from build123d import *

# Parameters (mm, degrees)
BOSS_EXTRUDE1_DEPTH        = 36.33
SKETCH2_R                  = 12.56
SKETCH2_R_2                = 9.25
BOSS_EXTRUDE2_DEPTH        = 20.17
SKETCH3_R                  = 13.815
BOSS_EXTRUDE3_DEPTH        = 20.35
BOSS_EXTRUDE4_DEPTH        = 47.86
CUT_EXTRUDE1_DEPTH         = 8.000000034
SKETCH6_R                  = 6.5
CUT_EXTRUDE2_DEPTH         = 86.564913353
SKETCH7_R                  = 3.8
BOSS_EXTRUDE5_DEPTH        = 17.8
F_10_32_TAPPED_HOLE1_D     = 4.0386
F_10_32_TAPPED_HOLE1_DEPTH = 17.8


with BuildPart() as part:
    # Sketch1 → Boss-Extrude1 (new body)
    with BuildSketch(Plane(origin=(0, 0, 0), x_dir=(1, 0, 0), z_dir=(0, 1, 0))):
        with BuildLine():
            Line((-25, 15), (-25, -15))
            ThreePointArc((-25, -15), (-0.303555948, -21.362892261), (25, -18.18))
            Line((25, -18.18), (25, 18.18))
            ThreePointArc((25, 18.18), (-0.303555948, 21.362892261), (-25, 15))
        make_face()
    extrude(amount=-BOSS_EXTRUDE1_DEPTH)

    # Sketch2 → Boss-Extrude2 (add)
    with BuildSketch(Plane(origin=(25, 0, 0), x_dir=(0, 0, -1), z_dir=(1, 0, 0))):
        with Locations((0, -18.165)):
            Circle(SKETCH2_R)
        with Locations((0, -18.165)):
            Circle(SKETCH2_R_2, mode=Mode.SUBTRACT)
    extrude(amount=BOSS_EXTRUDE2_DEPTH)

    # Sketch3 → Boss-Extrude3 (add)
    with BuildSketch(Plane.XZ.offset(36.33)):
        with Locations(Location((-1.315, 0, 0), (0, 0, 270))):
            Circle(SKETCH3_R)
    extrude(amount=BOSS_EXTRUDE3_DEPTH)

    # Sketch4 → Boss-Extrude4 (add)
    with BuildSketch(Plane(origin=(25, 0, 0), x_dir=(0, 0, -1), z_dir=(1, 0, 0))):
        Polygon((-9.13, -66), (-9.13, -53.08), (9.13, -53.08), (9.13, -66), (4.07, -71.38), (-4.07, -71.38), align=None)
    extrude(amount=-BOSS_EXTRUDE4_DEPTH)

    # Sketch5 → Cut-Extrude1 (cut)
    with BuildSketch(Plane(origin=(25, 0, 0), x_dir=(0, 0, -1), z_dir=(1, 0, 0))):
        Polygon((-9.13, -66), (-4.07, -71.38), (4.07, -71.38), (9.13, -66), (9.13, -53.08), (-9.13, -53.08), align=None)
    extrude(amount=-CUT_EXTRUDE1_DEPTH, mode=Mode.SUBTRACT)

    # Sketch6 → Cut-Extrude2 (cut, through all)
    with BuildSketch(Plane(origin=(16.999999966, 0, 0), x_dir=(0, 0, -1), z_dir=(1, 0, 0))):
        with Locations((0, -61.881671093)):
            Circle(SKETCH6_R)
    extrude(amount=-CUT_EXTRUDE2_DEPTH, mode=Mode.SUBTRACT)

    # Sketch7 → Boss-Extrude5 (add)
    with BuildSketch(Plane.XZ.offset(71.38)):
        with Locations(Location((-13.64, 12.01, 0), (0, 0, 270))):
            Circle(SKETCH7_R)
        with Locations(Location((8.41, -12.01, 0), (0, 0, 270))):
            Circle(SKETCH7_R)
    extrude(amount=-BOSS_EXTRUDE5_DEPTH)

    # #10-32 Tapped Hole1
    with Locations(Plane(origin=(0, -71.38, 0), x_dir=(-1, 0, 0), z_dir=(0, -1, 0))):
        with Locations((13.64, -12.01), (-8.41, 12.01)):
            Hole(F_10_32_TAPPED_HOLE1_D / 2, depth=F_10_32_TAPPED_HOLE1_DEPTH)


solid = part.part
Check sheet for the modelled part. Datum: model origin and axes. Units: mm. A direction names the side the tool comes from. Give positions to 0.01 mm unless a question says otherwise; leave off trailing zeros. Order: outer loops, then holes, each group sorted by start corner. A loop starts at its lowest first (then second) coordinate and runs counter-clockwise, first axis right, second up. Notation, with made-up numbers: (9, 38) - (42, 38) arc R23 cw to (42, 60) - close; hole circle Ø3 at (80.5, 33.25). An arc over 180 degrees is marked (long way). Answer as CSV lines item,"result".
1. Section check C-C (x = -13.64). Record the boundary of the cut face in (y, z).
Result sheet:
outline,"(-71.38, -4.07) - (-66, -9.13) - (-53.08, -9.13) - (-53.08, -6.24) - (-36.33, -6.24) - (-36.33, -19.17) - (0, -19.17) - (0, 19.17) - (-36.33, 19.17) - (-36.33, 6.24) - (-53.08, 6.24) - (-53.08, 9.13) - (-53.58, 9.13) - (-53.58, 9.99) - (-71.38, 9.99) - (-71.38, 8.21) - (-66.98, 8.21) - (-71.38, 4.07) - close; (-71.38, 14.03) - (-53.58, 14.03) - (-53.58, 15.81) - (-71.38, 15.81) - close; hole circle Ø13 at (-61.88, 0)"
2. Mould release check, pull along X, two halves, no side actions. Record for faces 1 (the face through (-11.714, -62.355, 11.403)), 2 (the face through (-25, -18, 0)), 3 (the face through (25, -18, 0)): released by +X, released by -X, zero draft, split by the parting line, or undercut.
Result sheet:
face 1,"undercut"
face 2,"released by -X"
face 3,"released by +X"
3. Section check D-D (z = -5). Record the boundary of the cut face in (x, y).
Result sheet:
outline,"(-25, -36.33) - (-14.19, -36.33) - (-14.19, -53.08) - (-22.86, -53.08) - (-22.86, -57.73) - (17, -57.73) - (17, -53.08) - (11.56, -53.08) - (11.56, -36.33) - (25, -36.33) - (25, -29.69) - (45.17, -29.69) - (45.17, -25.95) - (25, -25.95) - (25, -10.38) - (45.17, -10.38) - (45.17, -6.64) - (25, -6.64) - (25, 0) - (-25, 0) - close; (-22.86, -70.39) - (17, -70.39) - (17, -66.03) - (-22.86, -66.03) - close"
4. Section check B-B (x = 14). Record the boundary of the cut face in (y, z), then the cut area to 3 significant figures.
Result sheet:
outline,"(-71.38, -4.07) - (-66, -9.13) - (-53.08, -9.13) - (-53.08, 9.13) - (-66, 9.13) - (-71.38, 4.07) - close; (-36.33, -20.76) - (0, -20.76) - (0, 20.76) - (-36.33, 20.76) - close; hole circle Ø13 at (-61.88, 0)"
area,"1,680 mm²"
5. Scan lines: probe 1 along Y at (x, z) = (-21.5, 0.5); probe 2 along X at (y, z) = (-64, 12.01); probe 3 along Z at (x, y) = (-13.64, -60.75). Record each from-to range of solid material in increasing order. Write a range as from..to.
Result sheet:
probe 1,"-71.38..-68.36, -55.4..-53.08, -36.33..0"
probe 2,"-17.44..-15.66, -11.62..-9.84"
probe 3,"-9.13..-6.4, 6.4..9.99, 14.03..15.81"
6. Section check A-A (z = 0). Record the boundary of the cut face in (x, y) (3 decimals).
Result sheet:
outline,"(-25, -36.33) - (-15.13, -36.33) - (-15.13, -53.08) - (-22.86, -53.08) - (-22.86, -55.382) - (17, -55.382) - (17, -53.08) - (12.5, -53.08) - (12.5, -36.33) - (25, -36.33) - (25, -30.725) - (45.17, -30.725) - (45.17, -27.415) - (25, -27.415) - (25, -8.915) - (45.17, -8.915) - (45.17, -5.605) - (25, -5.605) - (25, 0) - (-25, 0) - close; (-22.86, -71.38) - (17, -71.38) - (17, -68.382) - (-22.86, -68.382) - close"
7. Go/stop test with flat-tipped pins: P1, Ø2, axis at x = -5.5, y = -31.5, coming from the -Z side; P2, Ø6.5, axis at x = 7, y = -58.5, coming from the +Z side; P3, Ø4, axis at x = -8, y = -60.5, coming from the -Z side. Record where each tip stops, or that it passes through.
Result sheet:
P1,"z = -20.97"
P2,"z = 12.62"
P3,"z = -9.13"
8. Tool access check on faces 4 (the face through (-0.7, -46.4, 13.8)), 5 (the face through (10, -53.58, -14)), 6 (the face through (25, -6, 4)), 7 (the face through (8.147, -62.355, -14.012)). Record the directions out of +Z, -Z, +X, -X, +Y, -Y that give a thin tool (end or side, any length) a straight path to the whole face; none if there is none.
Result sheet:
face 4,"none"
face 5,"-Z, +X"
face 6,"+X"
face 7,"-Y"
